The listing builds one solid part. Answer for the finished solid, in the listing's coordinates (mm). A direction names the side the tool comes from. Round coordinates to 2 decimals unless told otherwise and drop trailing zeros. Order: outer loops, then holes, each group sorted by start corner. A loop starts at its lowest first (then second) coordinate and runs counter-clockwise, first axis right, second up. Notation, with made-up numbers: M 89.25,73 L 120.25,73 A34 ccw 120.25,112 Z; hole C 6.5,82.5 d8. An arc over 180 degrees is marked long. Put each result on its own line as item: value. Start each with the question number.
1. The part is cut by section B-B (y = 0). Give the vertices of the cut face in (x, z).
2. The mould has two halves that part along Z. Classify faces 4 (the face through (-7.01, 1.5, 12.77)), 5 (the face through (7, -8, 12)), 6 (the face through (-6.5, 2, 3)), 7 (the face through (6.99, 1.5, 12.77)): +Z half, -Z half, draft (parallel to the pull), parting line (faces both ways), or undercut.
3. The part is cut by section D-D (z = 8). Give the vertices of the cut face in (x, y), then the cut area to 3 significant figures.
4. The part is cut by section C-C (y = 7). Give the vertices of the cut face in (x, z).
5. Consider line 1 (X direction, y = 5.25, z = 3.5); line 2 (Y direction, x = 7.2, z = 8); line 3 (Z direction, x = 4, y = 3.75). Determine where each line is inside the solid, lowest interval first.
6. Which of the six approach directions +Z, -Z, +X, -X, +Y, -Y give full straight-line access (tool end or side, diameter ignored) to faces 1 (the face through (7, 8, 12)), 2 (the face through (6.5, 2, 3)), 3 (the face through (7, 0, 14))?
7. The part is cut by section A-A (z = 4). Give the vertices of the cut face in (x, y), then the cut area to 3 significant figures.
8. Each of these flat-tipped pins is pushed along its axis until it touches: pin 1 Ø8 at (y, z) = (0, 8) entering from -X; pin 2 Ø3.5 at (x, y) = (2, -1) entering from +Z; pin 3 Ø3 at (x, y) = (5.5, 4) entering from +Z; pin 4 Ø7 at (y, z) = (-3, 11) entering from +X. Where does it stop, or does it pass through?
from build123d import *

# Parameters (mm, degrees)
SKETCH2_W                    = 15
SKETCH2_H                    = 18
BASE_FLANGE1_DEPTH           = 1
EDGE_FLANGE1_STRIP_W         = 5.4732
EDGE_FLANGE1_STRIP_H         = 1
EDGE_FLANGE1_STRIP_CUT_DEPTH = 18
EDGE_FLANGE1_DEPTH           = 18
EDGE_FLANGE2_STRIP_W         = 5.4732
EDGE_FLANGE2_STRIP_H         = 1
EDGE_FLANGE2_STRIP_CUT_DEPTH = 18
EDGE_FLANGE2_DEPTH           = 18
SKETCH13_R                   = 5
CUT_EXTRUDE1_DEPTH           = 24.043437244
FILLET1_R                    = 5


# Sheet-metal steps are written as plain solids
with BuildPart() as part:
    # Sketch2 → Base-Flange1 (new body)
    with BuildSketch(Plane.XY):
        Rectangle(SKETCH2_W, SKETCH2_H)
    extrude(amount=-BASE_FLANGE1_DEPTH)

    # Edge-Flange1 strip (across the edge) → Edge-Flange1 strip cut (cut)
    with BuildSketch(Plane(origin=(7.5, -9, 0), x_dir=(-1, 0, 0), z_dir=(0, 1, 0))):
        with Locations((-1, -0.5)):
            Rectangle(EDGE_FLANGE1_STRIP_W, EDGE_FLANGE1_STRIP_H)
    extrude(amount=EDGE_FLANGE1_STRIP_CUT_DEPTH, mode=Mode.SUBTRACT)

    # Edge-Flange1 section (across the edge) → Edge-Flange1 (add)
    with BuildSketch(Plane(origin=(7.5, -9, 0), x_dir=(-1, 0, 0), z_dir=(0, 1, 0))):
        with BuildLine():
            Line((0, 0.7366), (0, 14))
            Line((0, 14), (1, 14))
            Line((1, 14), (1, 0.7366))
            ThreePointArc((1, 0.7366), (1.215745145, 0.215745145), (1.7366, 0))
            Line((1.7366, 0), (1.7366, -1))
            ThreePointArc((1.7366, -1), (0.508638364, -0.491361636), (0, 0.7366))
        make_face()
    extrude(amount=EDGE_FLANGE1_DEPTH)

    # Edge-Flange2 strip (across the edge) → Edge-Flange2 strip cut (cut)
    with BuildSketch(Plane(origin=(-7.5, 9, 0), x_dir=(1, 0, 0), z_dir=(0, -1, 0))):
        with Locations((-1, -0.5)):
            Rectangle(EDGE_FLANGE2_STRIP_W, EDGE_FLANGE2_STRIP_H)
    extrude(amount=EDGE_FLANGE2_STRIP_CUT_DEPTH, mode=Mode.SUBTRACT)

    # Edge-Flange2 section (across the edge) → Edge-Flange2 (add)
    with BuildSketch(Plane(origin=(-7.5, 9, 0), x_dir=(1, 0, 0), z_dir=(0, -1, 0))):
        with BuildLine():
            Line((0, 0.7366), (0, 15))
            Line((0, 15), (1, 15))
            Line((1, 15), (1, 0.7366))
            ThreePointArc((1, 0.7366), (1.215745145, 0.215745145), (1.7366, 0))
            Line((1.7366, 0), (1.7366, -1))
            ThreePointArc((1.7366, -1), (0.508638364, -0.491361636), (0, 0.7366))
        make_face()
    extrude(amount=EDGE_FLANGE2_DEPTH)

    # Sketch13 → Cut-Extrude1 (cut, through all)
    with BuildSketch(Plane.ZY.offset(7.5)):
        with Locations((8, 0)):
            Circle(SKETCH13_R)
    extrude(amount=-CUT_EXTRUDE1_DEPTH, mode=Mode.SUBTRACT)

    # Fillet1
    fillet1_edges = [part.edges().sort_by_distance(p)[0] for p in [
        (7, -9, 14),
        (7, 9, 14),
        (-7, 9, 15),
        (-7, -9, 15),
    ]]
    fillet(fillet1_edges, radius=FILLET1_R)


solid = part.part
Resolved:
1. outline: M -7.5,0.74 A1.74 ccw -5.76,-1 L 5.76,-1 A1.74 ccw 7.5,0.74 L 7.5,3 L 6.5,3 L 6.5,0.74 A0.74 cw 5.76,0 L -5.76,0 A0.74 cw -6.5,0.74 L -6.5,3 L -7.5,3 Z; M -7.5,13 L -6.5,13 L -6.5,15 L -7.5,15 Z; M 6.5,13 L 7.5,13 L 7.5,14 L 6.5,14 Z
2. face 4: undercut
2. face 5: +Z half
2. face 6: draft
2. face 7: undercut
3. outline: M -7.5,-9 L -6.5,-9 L -6.5,-5 L -7.5,-5 Z; M -7.5,5 L -6.5,5 L -6.5,9 L -7.5,9 Z; M 6.5,-9 L 7.5,-9 L 7.5,-5 L 6.5,-5 Z; M 6.5,5 L 7.5,5 L 7.5,9 L 6.5,9 Z
3. area: 16.0 mm2
4. outline: M -7.5,0.74 A1.74 ccw -5.76,-1 L 5.76,-1 A1.74 ccw 7.5,0.74 L 7.5,13 L 6.5,13 L 6.5,0.74 A0.74 cw 5.76,0 L -5.76,0 A0.74 cw -6.5,0.74 L -6.5,14 L -7.5,14 Z
5. line 1: -7.5 to -6.5, 6.5 to 7.5
5. line 2: -9 to -5, 5 to 9
5. line 3: -1 to 0
6. face 1: +Z, +X, +Y
6. face 2: +Z, +Y, -Y
6. face 3: +Z, +X, +Y, -Y
7. outline: M -7.5,-9 L -6.5,-9 L -6.5,-3 L -7.5,-3 Z; M -7.5,3 L -6.5,3 L -6.5,9 L -7.5,9 Z; M 6.5,-9 L 7.5,-9 L 7.5,-3 L 6.5,-3 Z; M 6.5,3 L 7.5,3 L 7.5,9 L 6.5,9 Z
7. area: 24.0 mm2
8. pin 1: through
8. pin 2: z = 0
8. pin 3: z = 14
8. pin 4: x = 7.5
